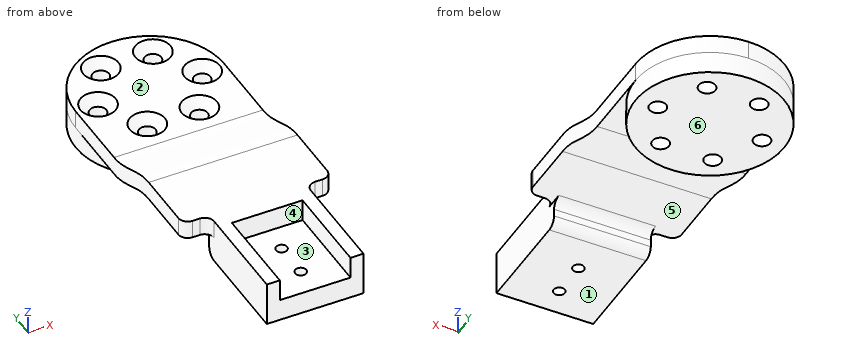
from build123d import *

# Parameters (mm, degrees)
SKETCH7_W           = 40
SKETCH7_H           = 40
BOSS_EXTRUDE1_DEPTH = 11
LOFT1_START         = -20
LOFT1_DEPTH         = 40
SKETCH16_W          = 49.026286786
SKETCH16_H          = 65.242270374
SKETCH16_R          = 20
CUT_EXTRUDE3_DEPTH  = 6
SKETCH17_W          = 40
SKETCH17_H          = 5
BOSS_EXTRUDE5_DEPTH = 18
SKETCH10_R          = 2.25
CUT_EXTRUDE1_DEPTH  = 25
CHAMFER1_SIZE       = 2.5
FILLET3_R           = 20
SKETCH11_W          = 26
SKETCH11_H          = 12
BOSS_EXTRUDE6_DEPTH = 30
SKETCH21_W          = 19
SKETCH21_H          = 6
CUT_EXTRUDE4_DEPTH  = 25
FILLET5_R           = 2.5
FILLET7_R           = 2.5
SKETCH22_R          = 1.5
CUT_EXTRUDE5_DEPTH  = 12.5


# Read off the part's stored shape, not the designer's step: Loft1
with BuildPart() as part:
    # Sketch7 → Boss-Extrude1 (new body)
    with BuildSketch(Plane.XY):
        Rectangle(SKETCH7_W, SKETCH7_H)
    extrude(amount=BOSS_EXTRUDE1_DEPTH)

    # Loft1 outline → Loft1 (add)
    with BuildSketch(Plane.YZ.offset(LOFT1_START)):
        with BuildLine():
            add(Edge.make_bspline(
                [(-38, 16), (-31.772819436, 16), (-26.227180564, 11), (-20, 11)],
                knots=[0, 0, 0, 0, 1, 1, 1, 1], degree=3))
            Line((-38, 16), (-38, 11))
            add(Edge.make_bspline(
                [(-38, 11), (-31.772819436, 11), (-26.227180564, 6), (-20, 6)],
                knots=[0, 0, 0, 0, 1, 1, 1, 1], degree=3))
            Line((-20, 6), (-20, 11))
        make_face()
    extrude(amount=LOFT1_DEPTH)

    # Sketch16 → Cut-Extrude3 (cut)
    with BuildSketch(Plane(origin=(0, 0, 0), x_dir=(-1, 0, 0), z_dir=(0, 0, -1))):
        Rectangle(SKETCH16_W, SKETCH16_H)
        Circle(SKETCH16_R, mode=Mode.SUBTRACT)
    extrude(amount=-CUT_EXTRUDE3_DEPTH, mode=Mode.SUBTRACT)

    # Sketch17 → Boss-Extrude5 (add)
    with BuildSketch(Plane(origin=(0, -38, 0), x_dir=(-1, 0, 0), z_dir=(0, -1, 0))):
        with Locations((0, -13.5)):
            Rectangle(SKETCH17_W, SKETCH17_H)
    extrude(amount=BOSS_EXTRUDE5_DEPTH)

    # Sketch10 → Cut-Extrude1 (cut)
    with BuildSketch(Plane.XY.offset(11)):
        with Locations((-7.00009521, 12.124420806)):
            Circle(SKETCH10_R)
        with Locations((6.99990479, 12.124420806)):
            Circle(SKETCH10_R)
        with Locations((13.99990479, 6.5153e-05)):
            Circle(SKETCH10_R)
        with Locations((6.99990479, -12.1242905)):
            Circle(SKETCH10_R)
        with Locations((-7.00009521, -12.1242905)):
            Circle(SKETCH10_R)
        with Locations((-14.00009521, 6.5153e-05)):
            Circle(SKETCH10_R)
    extrude(amount=-CUT_EXTRUDE1_DEPTH, mode=Mode.SUBTRACT)

    # Chamfer1
    chamfer1_edges = [part.edges().sort_by_distance(p)[0] for p in [
        (4.74990479, 12.124420806, 11),
        (-9.25009521, 12.124420806, 11),
        (-16.25009521, 6.5153e-05, 11),
        (-9.25009521, -12.1242905, 11),
        (4.74990479, -12.1242905, 11),
        (11.74990479, 6.5153e-05, 11),
    ]]
    chamfer(chamfer1_edges, length=CHAMFER1_SIZE)

    # Fillet3
    fillet3_edges = [part.edges().sort_by_distance(p)[0] for p in [
        (20, 20, 8.5),
        (-20, 20, 8.5),
    ]]
    fillet(fillet3_edges, radius=FILLET3_R - 0.0001)  # a hair under: the kernel refuses the full size

    # Sketch11 → Boss-Extrude6 (add)
    with BuildSketch(Plane(origin=(0, -56, -3.472963553), x_dir=(1, 0, 0), z_dir=(0, 1, 0))):
        with Locations((0, -13.472963553)):
            Rectangle(SKETCH11_W, SKETCH11_H)
    extrude(amount=-BOSS_EXTRUDE6_DEPTH)

    # Sketch21 → Cut-Extrude4 (cut)
    with BuildSketch(Plane(origin=(0, -86, 0), x_dir=(-1, 0, 0), z_dir=(0, -1, 0))):
        with Locations((0, -13)):
            Rectangle(SKETCH21_W, SKETCH21_H)
    extrude(amount=-CUT_EXTRUDE4_DEPTH, mode=Mode.SUBTRACT)

    # Fillet5
    fillet5_edges = [part.edges().sort_by_distance(p)[0] for p in [
        (-13, -56, 13.5),
        (-20, -56, 13.5),
        (13, -56, 13.5),
        (20, -56, 13.5),
    ]]
    fillet(fillet5_edges, radius=FILLET5_R)

    # Fillet7
    fillet7_edges = [part.edges().sort_by_distance(p)[0] for p in [
        (0, -56, 11),
        (0, -56, 4),
    ]]
    fillet(fillet7_edges, radius=FILLET7_R)

    # Sketch22 → Cut-Extrude5 (cut, symmetric)
    with BuildSketch(Plane.XY):
        with Locations(Location((0, -68.5, 0), (0, 0, 180))):
            Circle(SKETCH22_R)
        with Locations(Location((0, -78.5, 0), (0, 0, 180))):
            Circle(SKETCH22_R)
    extrude(amount=CUT_EXTRUDE5_DEPTH, both=True, mode=Mode.SUBTRACT)


solid = part.part
Part model, mm, in its own coordinate system. Face numbers are marked on the shaded views. A direction names the side the tool comes from. Coordinates: 2 decimals unless noted, no trailing zeros. Loops run counter-clockwise (first coordinate to the right, second up) from the corner with the lowest first, then second, coordinate; pieces in that order, holes last. Notation, with made-up numbers: (17.5, 50.5) - (71.5, 50.5) arc R6 ccw to (71.5, 61.5) - close; hole circle Ø5 at (67.25, -30). An arc over 180 degrees is marked (long way). Write each question's results on one line, items separated by ' | '. Start each with the question number.
Q1. Two-plate mould, pull along Y, no slides. Class the marked faces 4, 5 and 6: +Y half, -Y half, draft (parallel to the pull), parting line (faces both ways), or undercut.
Q2. Which spindle directions (+Z, -Z, +X, -X, +Y, -Y) get a long thin tool onto all of the face, cutting with end or side? Do the marked faces 1, 2 and 3. Say none if no direction does.
Q3. Drop flat-ended pins along their axis: pin 1 Ø5 at (x, y) = (0, -78.5) entering from -Z; pin 2 Ø2 at (x, z) = (-16, 13) entering from -Y; pin 3 Ø3.5 at (y, z) = (-62.5, 10) entering from +X. Give the stop position or say it passes through.
Q4. Slice it at B-B on y = -55. Give the cut face in (x, z).
Q5. Probe line 1 along X through (y, z) = (-63, 10.5); line 2 along Y through (x, z) = (0, 5.5); line 3 along X through (y, z) = (-2, 6.75). List the from-to ranges inside material, lowest first.
Q6. Slice it at A-A on y = -78.5. Give the cut face in (x, z).
Answer:
1) face 4: -Y half | face 5: undercut | face 6: draft
2) face 1: -Z, +X, -X, -Y | face 2: +Z, +X, -X, +Y | face 3: +Z, -Y
3) pin 1: stops at z = 4 | pin 2: stops at y = -56.05 | pin 3: stops at x = 13
4) outline: (-19.5, 11) - (-13, 11) - (-13, 10.5) - (13, 10.5) - (13, 11) - (19.5, 11) - (19.5, 16) - (-19.5, 16) - close
5) line 1: x = -13 to -9.5, 9.5 to 13 | line 2: y = -86 to -80, -77 to -70, -67 to -56.21, -20 to 20 | line 3: x = -20 to -15.03, -12.97 to 12.97, 15.03 to 20
6) outline: (-13, 4) - (-1.5, 4) - (-1.5, 10) - (-9.5, 10) - (-9.5, 16) - (-13, 16) - close; (1.5, 4) - (13, 4) - (13, 16) - (9.5, 16) - (9.5, 10) - (1.5, 10) - close
